Can you work these out from the drawing? Everything is in mm from the part's minimum corner. Round coordinates to 2 decimals unless told otherwise and drop trailing zeros. Write each loop counter-clockwise with the first axis right and the second up, starting at its lowest first coordinate (ties: lowest second). Pieces come first, ordered by that corner, then holes. Notation, with made-up numbers: M -34.5,15.5 L -25.5,15.5 A24 cw -25.5,37.5 Z; hole C 89,60 d4. An arc over 180 degrees is marked long. Answer in a Markdown table with one row per item. Add a question column.
(1) I'm going to push flat-ended pins straight in: pin 1 (3 mm diameter, centred on x = 62, z = 6, fed in from -Y); pin 2 (6 mm diameter, centred on x = 35.5, z = 11, fed in from +Y). Where does each tip first touch, or does it pass through?
(2) Suppose I cut it at B-B, the plane z = 10.25. Write out the boundary of the cut face in (x, y), then the cut area to 3 significant figures.
(3) If I drill on probe 1 along Y at (x, z) = (83, 10.25) (1 decimal); probe 2 along Y at (x, z) = (96.5, 15), over which ranges is the centre line in solid material (lowest first)?
(4) Suppose I cut it at A-A, the plane x = 63.5. Write out the boundary of the cut face in (y, z).
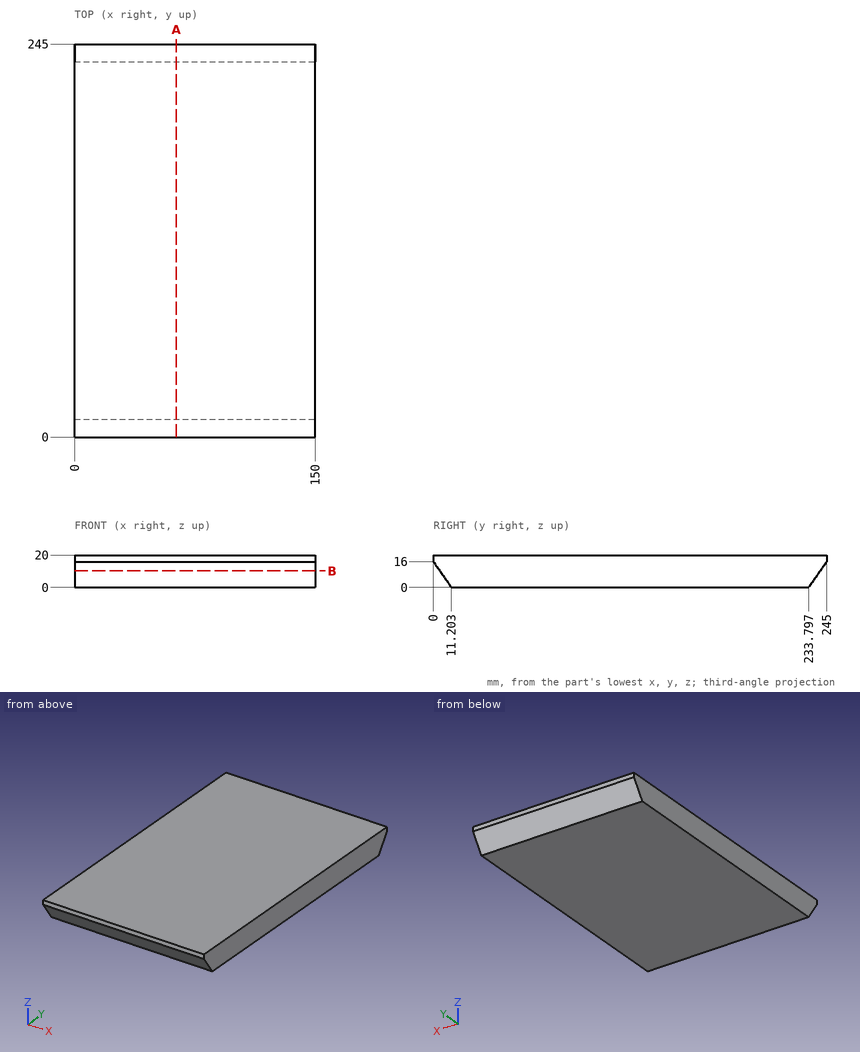
Calculated:
| question | item | result |
|---|---|---|
| 1 | pin 1 | y = 5.95 |
| 1 | pin 2 | y = 243.6 |
| 2 | outline | M 0,4.03 L 150,4.03 L 150,240.97 L 0,240.97 Z |
| 2 | area | 35,500 mm² |
| 3 | probe 1 | 4 to 241 |
| 3 | probe 2 | 0.7 to 244.3 |
| 4 | outline | M 0,16 L 11.2,0 L 233.8,0 L 245,16 L 245,20 L 0,20 Z |
